The model under review builds one solid part; all positions refer to its coordinate system, in mm. Face numbers are marked on the shaded views. A direction names the side the tool comes from. Round coordinates to 2 decimals unless told otherwise and drop trailing zeros. Write each loop counter-clockwise with the first axis right and the second up, starting at its lowest first coordinate (ties: lowest second). Pieces come first, ordered by that corner, then holes. Notation, with made-up numbers: (-14.75, 11.5) - (14.25, 11.5) arc R21 cw to (14.25, 27.5) - close; hole circle Ø5 at (73.5, 42.25). An arc over 180 degrees is marked (long way). Return JSON: item names as keys, results as strings.
from build123d import *

# Parameters (mm, degrees)
F0_R     = 25
F1_DEPTH = 10


with BuildPart() as f1:
    # F0 (on Top) → F1 (new body)
    with BuildSketch(Plane.XY):
        Circle(F0_R)
        Polygon((-1.3539496528, -8.1774380319), (-4.9288194444, -8.1774380319), (-9.0091145833, -1.7102071291), (-13.0930989583, -8.1774380319), (-16.6901041667, -8.1774380319), (-11.0640190972, 0.3668328015), (-16.2178819444, 8.0662685653), (-12.6208767361, 8.0662685653), (-9.0091145833, 2.3258171765), (-5.4010416667, 8.0662685653), (-1.8298611111, 8.0662685653), (-6.7623697917, 0.3668328015), align=None, mode=Mode.SUBTRACT)
        with BuildLine():
            add(Edge.make_bspline(
                [(4.4731987847, -4.2557800458), (5.6998697917, -5.7314744902), (8.0167100694, -5.7314744902)],
                knots=[0, 0, 0, 1, 1, 1], degree=2))
            add(Edge.make_bspline(
                [(8.0167100694, -5.7314744902), (11.0972222222, -5.7314744902), (12.2962239583, -2.6435838652)],
                knots=[0, 0, 0, 1, 1, 1], degree=2))
            Line((12.2962239583, -2.6435838652), (15.2586805556, -3.7614224069))
            add(Edge.make_bspline(
                [(15.2586805556, -3.7614224069), (14.3031684028, -6.1151550458), (12.451171875, -7.2625074763)],
                knots=[0, 0, 0, 1, 1, 1], degree=2))
            add(Edge.make_bspline(
                [(12.451171875, -7.2625074763), (10.5991753472, -8.4098599069), (8.0167100694, -8.4098599069)],
                knots=[0, 0, 0, 1, 1, 1], degree=2))
            add(Edge.make_bspline(
                [(8.0167100694, -8.4098599069), (4.0987413194, -8.4098599069), (1.9608289931, -6.188939768)],
                knots=[0, 0, 0, 1, 1, 1], degree=2))
            add(Edge.make_bspline(
                [(1.9608289931, -6.188939768), (-0.1770833333, -3.9680196291), (-0.1770833333, 0.020044607)],
                knots=[0, 0, 0, 1, 1, 1], degree=2))
            add(Edge.make_bspline(
                [(-0.1770833333, 0.020044607), (-0.1770833333, 4.0191765515), (1.8851996528, 6.1644673501)],
                knots=[0, 0, 0, 1, 1, 1], degree=2))
            add(Edge.make_bspline(
                [(1.8851996528, 6.1644673501), (3.9474826389, 8.3097581487), (7.869140625, 8.3097581487)],
                knots=[0, 0, 0, 1, 1, 1], degree=2))
            add(Edge.make_bspline(
                [(7.869140625, 8.3097581487), (10.7282986111, 8.3097581487), (12.5268012153, 7.1624057181)],
                knots=[0, 0, 0, 1, 1, 1], degree=2))
            add(Edge.make_bspline(
                [(12.5268012153, 7.1624057181), (14.3253038194, 6.0150532876), (15.0520833333, 3.7904439126)],
                knots=[0, 0, 0, 1, 1, 1], degree=2))
            Line((15.0520833333, 3.7904439126), (12.052734375, 2.9714334959))
            add(Edge.make_bspline(
                [(12.052734375, 2.9714334959), (11.6727430556, 4.1925706487), (10.5604383681, 4.9138163084)],
                knots=[0, 0, 0, 1, 1, 1], degree=2))
            add(Edge.make_bspline(
                [(10.5604383681, 4.9138163084), (9.4481336806, 5.6350619681), (7.9392361111, 5.6350619681)],
                knots=[0, 0, 0, 1, 1, 1], degree=2))
            add(Edge.make_bspline(
                [(7.9392361111, 5.6350619681), (5.6334635417, 5.6350619681), (4.4399956597, 4.2054829751)],
                knots=[0, 0, 0, 1, 1, 1], degree=2))
            add(Edge.make_bspline(
                [(4.4399956597, 4.2054829751), (3.2465277778, 2.775903982), (3.2465277778, 0.020044607)],
                knots=[0, 0, 0, 1, 1, 1], degree=2))
            add(Edge.make_bspline(
                [(3.2465277778, 0.020044607), (3.2465277778, -2.7800856013), (4.4731987847, -4.2557800458)],
                knots=[0, 0, 0, 1, 1, 1], degree=2))
        make_face(mode=Mode.SUBTRACT)
    extrude(amount=F1_DEPTH)


solid = f1.part
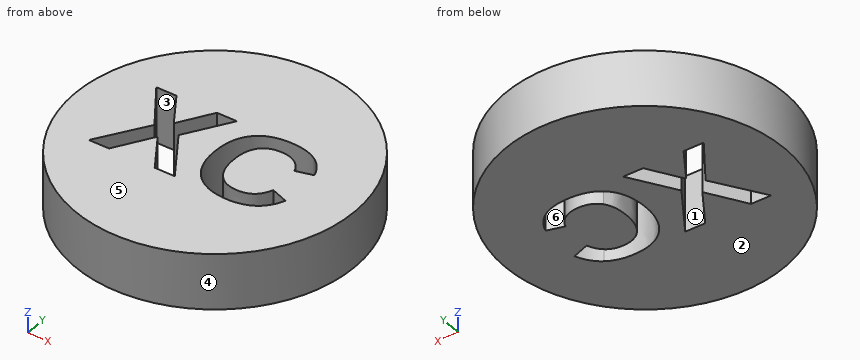
(1) Clearance check with flat-ended pins moving along their axes: pin 1 Ø4 at (x, z) = (-15, 7) entering from -Y; pin 2 Ø1 at (y, z) = (1, 7) entering from +X (3 decimals); pin 3 Ø3 at (x, z) = (-4, 5.5) entering from -Y. State where each tip first meets the part, or that it passes through.
Filled in:
{"pin 1": "stops at y = -21.35", "pin 2": "stops at x = 24.995", "pin 3": "stops at y = -24.87"}
(2) Wall thickness on line 1 (X direction, y = 6, z = 4); line 2 (X direction, y = -2.5, z = 4); line 3 (Y direction, x = 6, z = 7.5): over which ranges is each line inside the solid? List them lowest first.
Filled in:
{"line 1": "x = -24.27 to -14.83, -11.32 to -6.7, -3.15 to 1.73, 13.86 to 24.27", "line 2": "x = -24.87 to -12.95, -9.51 to -8.51, -4.95 to 0.07, 3.57 to 24.87", "line 3": "y = -24.27 to -8.24, -5.37 to 5.31, 8.17 to 24.27"}
(3) Add section A-A (x = -14.5). Write out the cut boundary in (y, z), plus the area to 3 significant figures.
Filled in:
{"outline": "(-20.37, 0) - (-8.18, 0) - (-8.18, 10) - (-20.37, 10) - close; (-4.85, 0) - (5.5, 0) - (5.5, 10) - (-4.85, 10) - close; (8.07, 0) - (20.37, 0) - (20.37, 10) - (8.07, 10) - close", "area": "348 mm2"}
(4) Add section D-D (y = 15). Write out the cut boundary in (x, z).
Filled in:
{"outline": "(-20, 0) - (20, 0) - (20, 10) - (-20, 10) - close"}
(5) For the marked faces 5 and 6, list the 3-axis set-ups (+Z, -Z, +X, -X, +Y, -Y) from which the entire face can be reached by the end or side of a thin tool; tool diameter is ignored.
Filled in:
{"face 5": "+Z, +X, -X, +Y, -Y", "face 6": "+Z, -Z"}
(6) Mouldability with a two-part tool opening along Y and no side actions: class the marked faces 1, 2, 3 and 4 as released by +Y, released by -Y, zero draft, split by the parting line, or undercut.
Filled in:
{"face 1": "undercut", "face 2": "zero draft", "face 3": "undercut", "face 4": "split by the parting line"}
(7) Add section B-B (z = 9.25). Give the number of separate pieces and of enclosed holes in the cut face, plus the area to 3 significant figures.
Filled in:
{"separate pieces": "1", "enclosed holes": "2", "area": "1,740 mm2"}
(8) Add section C-C (x = -3.5). Write out the cut boundary in (y, z), plus the area to 3 significant figures.
Filled in:
{"outline": "(-24.75, 0) - (-8.18, 0) - (-8.18, 10) - (-24.75, 10) - close; (-4.79, 0) - (5.46, 0) - (5.46, 10) - (-4.79, 10) - close; (8.07, 0) - (24.75, 0) - (24.75, 10) - (8.07, 10) - close", "area": "435 mm2"}
